Can you work these out from the model? Positions are in its coordinate system, mm. Face numbers are marked on the shaded views. A direction names the side the tool comes from. Give positions to 0.01 mm unless a question says otherwise; leave off trailing zeros. Order: outer loops, then holes, each group sorted by start corner. A loop starts at its lowest first (then second) coordinate and runs counter-clockwise, first axis right, second up. Notation, with made-up numbers: M 65.5,-38.5 L 86.5,-38.5 A16 ccw 86.5,-23.5 Z; hole C -7.75,17 d2. An arc over 180 degrees is marked long. One line per question, with ' | ' between items. Start each with the question number.
1) I'm going to push flat-ended pins straight in: pin 1 Ø4 at (x, z) = (-9, 7.5) entering from +Y; pin 2 Ø3.5 at (y, z) = (-30, 9.5) entering from +X. Where does each tip first touch, or does it pass through?
2) Please list where these lines run through material, in increasing order: line 1 along X through (y, z) = (-28.5, 12.5); line 2 along X through (y, z) = (-33.25, 2.25); line 3 along X through (y, z) = (-33.75, 8.75). Write a range as [from, to].
3) Thinking about a two-plate mould opening in Y: for the marked faces 6, 7, 8 and 9, which applies, +Y half, -Y half, draft (parallel to the pull), parting line (faces both ways), or undercut?
4) If we section it at A-A, the plane z = 8.5: Please give me the cut outline in (x, y).
5) If we section it at B-B, the plane x = -27.5: Please give me the cut outline in (y, z).
6) If we section it at C-C, the plane y = -29.25: Please give me the cut outline in (x, z), plus the area to 3 significant figures.
7) For the marked faces 1, 2, 3, 4 and 5, which set-ups out of +Z, -Z, +X, -X, +Y, -Y let a thin tool reach every point of the face, with its end or its side?
8) If we section it at D-D, the plane x = 4.5: Please give me the cut outline in (y, z).
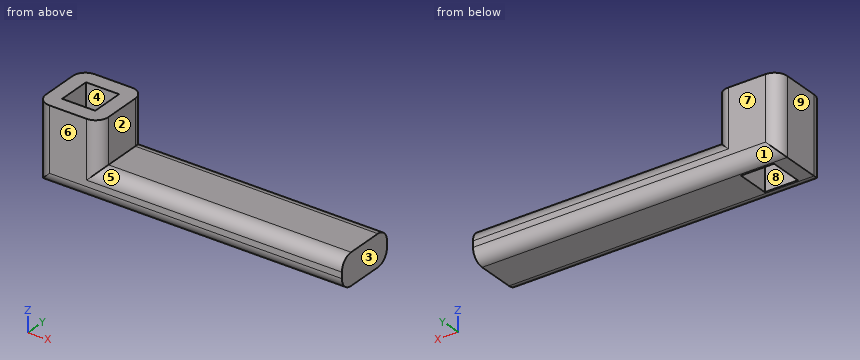
```python
from build123d import *

# Parameters (mm, degrees)
F0_W     = 47.7
F0_H     = 12.3
F1_DEPTH = 6.2
F0_W_2   = 12.3
F0_W_3   = 6.5
F0_H_2   = 6.5
F2_DEPTH = 15
F3_R     = 2.5


with BuildPart() as f1:
    # F0 (on Top) → F1 (new body)
    with BuildSketch(Plane.XY):
        with Locations((2.515334, -30.180186)):
            Rectangle(F0_W, F0_H)
    extrude(amount=F1_DEPTH)

    # F0 (on Top) → F2 (join)
    with BuildSketch(Plane.XY):
        with Locations((-27.484666, -30.180186)):
            Rectangle(F0_W_2, F0_H)
        with Locations((-27.484666, -30.180186)):
            Rectangle(F0_W_3, F0_H_2, mode=Mode.SUBTRACT)
    extrude(amount=F2_DEPTH)

    # F3
    f3_edges = [f1.edges().sort_by_distance(p)[0] for p in [
        (2.515334, -36.330186, 6.2),
        (2.515334, -24.030186, 6.2),
        (-3.634666, -24.030186, 0),
        (-3.634666, -36.330186, 0),
        (-33.634666, -36.330186, 7.5),
        (-21.334666, -36.330186, 10.6),
        (-21.334666, -24.030186, 10.6),
        (-33.634666, -24.030186, 7.5),
    ]]
    fillet(f3_edges, radius=F3_R)


solid = f1.part
```
Results found:
1) pin 1: stops at y = -24.8 | pin 2: stops at x = -21.33
2) line 1: x = [-33.63, -30.73], [-24.23, -21.33] | line 2: x = [-33.63, -30.73], [-24.23, 26.37] | line 3: x = [-33.63, -21.33]
3) face 6: -Y half | face 7: +Y half | face 8: undercut | face 9: draft
4) outline: M -33.63,-33.83 A2.5 ccw -31.13,-36.33 L -23.83,-36.33 A2.5 ccw -21.33,-33.83 L -21.33,-26.53 A2.5 ccw -23.83,-24.03 L -31.13,-24.03 A2.5 ccw -33.63,-26.53 Z; hole M -30.73,-33.43 L -24.23,-33.43 L -24.23,-26.93 L -30.73,-26.93 Z
5) outline: M -36.33,2.5 A2.5 ccw -33.83,0 L -33.43,0 L -33.43,15 L -36.33,15 Z; M -26.93,0 L -26.53,0 A2.5 ccw -24.03,2.5 L -24.03,15 L -26.93,15 Z
6) outline: M -33.63,0 L -30.73,0 L -30.73,15 L -33.63,15 Z; M -24.23,0 L 26.37,0 L 26.37,6.2 L -21.33,6.2 L -21.33,15 L -24.23,15 Z | area: 383 mm²
7) face 1: -Z, +X, -X, +Y | face 2: +Z, +X, +Y, -Y | face 3: +Z, -Z, +X, +Y, -Y | face 4: +Z, -Z | face 5: +Z, +X, -Y
8) outline: M -36.33,2.5 A2.5 ccw -33.83,0 L -26.53,0 A2.5 ccw -24.03,2.5 L -24.03,3.7 A2.5 ccw -26.53,6.2 L -33.83,6.2 A2.5 ccw -36.33,3.7 Z
